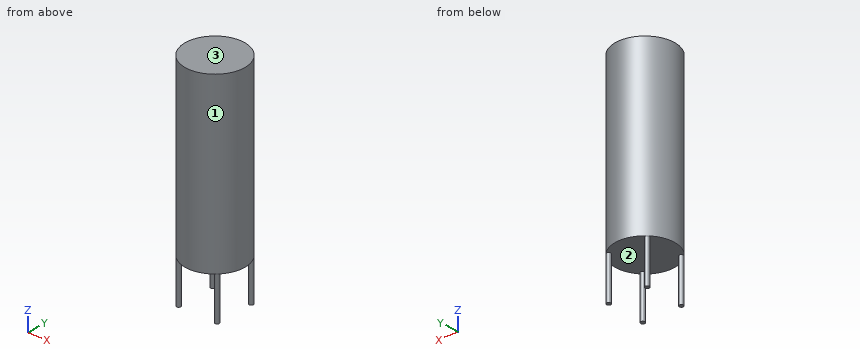
```python
from build123d import *

# Parameters (mm, degrees)
F0_R     = 2.5
F1_DEPTH = 50
F2_R     = 34.3198051534
F3_DEPTH = 200


# Not quite as in the source:
# - a feature of the source that left no trace in its solid (it failed there, or was rolled back) is left out


with BuildPart() as f1:
    # F0 (on Top) → F1 (new body)
    with BuildSketch(Plane.XY):
        with Locations((0, 45)):
            Circle(F0_R)
    extrude(amount=F1_DEPTH)



with BuildPart() as f1b:
    # F0 (on Top) → F1, piece 2 (new body)
    with BuildSketch(Plane.XY):
        with Locations((45, 45)):
            Circle(F0_R)
    extrude(amount=F1_DEPTH)


with BuildPart() as f1c:
    # F0 (on Top) → F1, piece 3 (new body)
    with BuildSketch(Plane.XY):
        Circle(F0_R)
    extrude(amount=F1_DEPTH)


with BuildPart() as f1d:
    # F0 (on Top) → F1, piece 4 (new body)
    with BuildSketch(Plane.XY):
        with Locations((45, 0)):
            Circle(F0_R)
    extrude(amount=F1_DEPTH)


with BuildPart() as f1_1:
    add(f1.part)

    add(f1b.part)  # F3 merges F1b

    add(f1c.part)  # F3 merges F1c

    add(f1d.part)  # F3 merges F1d
    # F2 (on face) → F3 (join)
    with BuildSketch(Plane.XY.offset(50)):
        with Locations((22.5, 22.5)):
            Circle(F2_R)
    extrude(amount=F3_DEPTH)


solid = f1_1.part
```
Work out the finished part from the listing and answer in its coordinate system (mm). Face numbers are marked on the shaded views. Round coordinates to 2 decimals unless told otherwise and drop trailing zeros. Write each loop counter-clockwise with the first axis right and the second up, starting at its lowest first coordinate (ties: lowest second). Pieces come first, ordered by that corner, then holes.
1) A cutting plane is placed at A-A on z = 27.5. Determine the outline of the cut face in (x, y), and give its area (3 significant figures).
2) A cutting plane is placed at B-B on x = 22.5. Determine the outline of the cut face in (y, z), and give its area (3 significant figures).
3) A cutting plane is placed at D-D on z = 172. Determine the outline of the cut face in (x, y).
4) Flat-ended cylindrical pins translate along their axes: P1, Ø1.5, axis at x = 3.5, y = 37.5, coming from the -Z side; P2, Ø4, axis at x = -3, z = 166, coming from the +Y side; P3, Ø6, axis at x = 10, z = 106, coming from the +Y side. Find the tip coordinate at first contact, or state that the pin passes through.
5) A cutting plane is placed at C-C on y = 51. Determine the outline of the cut face in (x, z), and give its area (3 significant figures).
6) Determine the mould class of the marked faces 1, 2 and 3 for opening direction X: pulls with the +X half, pulls with the -X half, needs draft (parallel to the pull), parting line crosses it, or undercut.
7) Consider probe 1 along Z at (x, y) = (33.5, 37); probe 2 along Y at (x, z) = (0, 23); probe 3 along X at (y, z) = (16, 237.5). Determine where each line is inside the solid, lowest interval first.
Entries:
1. outline: circle Ø5 at (0, 0); circle Ø5 at (0, 45); circle Ø5 at (45, 0); circle Ø5 at (45, 45)
1. area: 78.5 mm2
2. outline: (-11.82, 50) - (56.82, 50) - (56.82, 250) - (-11.82, 250) - close
2. area: 13,700 mm2
3. outline: circle Ø68.64 at (22.5, 22.5)
4. P1: stops at z = 50
4. P2: stops at y = 47.51
4. P3: stops at y = 55.48
5. outline: (3.38, 50) - (41.62, 50) - (41.62, 250) - (3.38, 250) - close
5. area: 7,650 mm2
6. face 1: parting line crosses it
6. face 2: undercut
6. face 3: needs draft
7. probe 1: z = 50 to 250
7. probe 2: y = -2.5 to 2.5, 42.5 to 47.5
7. probe 3: x = -11.2 to 56.2
